Could you check a few things on this model? Use its own coordinates, in mm. Face numbers are marked on the shaded views. A direction names the side the tool comes from. Coordinates: 2 decimals unless noted, no trailing zeros. Loops run counter-clockwise (first coordinate to the right, second up) from the corner with the lowest first, then second, coordinate; pieces in that order, holes last. Notation, with made-up numbers: (1, 61) -> (59, 61) arc R37 ccw to (59, 98) -> close; hole circle Ø3 at (11.25, 64). An arc over 180 degrees is marked (long way). One line per question, with ' | ' between items.
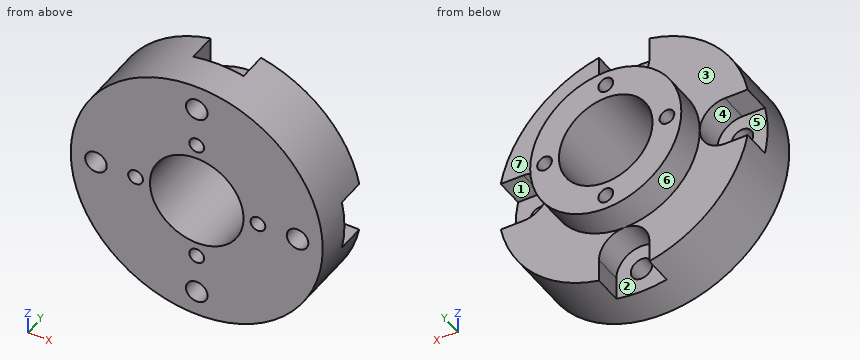
```python
from build123d import *

# Parameters (mm, degrees)
HOLE_WIZARD_4_1_4_1_1_D     = 4.1
HOLE_WIZARD_4_1_4_1_1_DEPTH = 26.501
HOLE_WIZARD_6_0_6_1_D       = 6
HOLE_WIZARD_6_0_6_1_DEPTH   = 18.001
CUT_EXTRUDE_1_DEPTH         = 8
PATTERN_CIRCULAR_1_COUNT    = 4


with BuildPart() as part:
    # Эскиз1 → Повернуть1 (revolve)
    with BuildSketch(Plane.XY):
        Polygon((-13, 0), (-13, 26.5), (-21, 26.5), (-21, 18), (-35, 18), (-35, 0), align=None)
    revolve(axis=Axis((0, 0, 0), (0, 1, 0)))

    # Диаметр отверстия Ø4.1 (4.1)1
    with Locations(Plane(origin=(0, 26.5, 0), x_dir=(1, 0, 0), z_dir=(0, 1, 0))):
        with Locations((17, 0)):
            hole_wizard_4_1_4_1_1 = Hole(HOLE_WIZARD_4_1_4_1_1_D / 2, depth=HOLE_WIZARD_4_1_4_1_1_DEPTH)

    # Диаметр отверстия Ø6.0 (6)1
    with Locations(Plane(origin=(0, 18, 0), x_dir=(1, 0, 0), z_dir=(0, 1, 0))):
        with Locations((28, 0)):
            hole_wizard_6_0_6_1 = Hole(HOLE_WIZARD_6_0_6_1_D / 2, depth=HOLE_WIZARD_6_0_6_1_DEPTH)

    # Эскиз4 → Вырез-Вытянуть1 (cut)
    with BuildSketch(Plane(origin=(0, 18, 0), x_dir=(1, 0, 0), z_dir=(0, 1, 0))):
        with BuildLine():
            Line((28, 7), (48, 7))
            Line((48, 7), (48, -7))
            Line((48, -7), (28, -7))
            ThreePointArc((28, -7), (21, 0), (28, 7))
        make_face()
    cut_extrude_1 = extrude(amount=-CUT_EXTRUDE_1_DEPTH, mode=Mode.SUBTRACT)

    # Круговой массив1: Диаметр отверстия Ø4.1 (4.1)1, Диаметр отверстия Ø6.0 (6)1, Вырез-Вытянуть1 ×4 about axis
    pattern_circular_1_axis = Axis((0, 0, 0), (0, 1, 0))
    for i in range(1, PATTERN_CIRCULAR_1_COUNT):
        add(hole_wizard_4_1_4_1_1.rotate(pattern_circular_1_axis, i * 360 / PATTERN_CIRCULAR_1_COUNT), mode=Mode.SUBTRACT)
        add(hole_wizard_6_0_6_1.rotate(pattern_circular_1_axis, i * 360 / PATTERN_CIRCULAR_1_COUNT), mode=Mode.SUBTRACT)
        add(cut_extrude_1.rotate(pattern_circular_1_axis, i * 360 / PATTERN_CIRCULAR_1_COUNT), mode=Mode.SUBTRACT)


solid = part.part
```
Q1. We'd pull the mould along Z, two halves only. Please class the marked faces 5, 6 and 7: released by +Z, released by -Z, zero draft, split by the parting line, or undercut.
Values follow:
face 5: undercut | face 6: split by the parting line | face 7: zero draft
Q2. Imagine slicing it at A-A on y = 2.75. Give the number of separate pieces and of enclosed holes in the cut face, plus the area to 3 significant figures.
Values follow:
separate pieces: 1 | enclosed holes: 9 | area: 3,150 mm2
Q3. For pin 1 (4 mm diameter, centred on x = 30.5, z = 2, fed in from +Y); pin 2 (3 mm diameter, centred on x = 32, y = 14.5, fed in from -Z); pin 3 (3 mm diameter, centred on x = -31.5, y = 15, fed in from -Z); pin 4 (3.5 mm diameter, centred on x = 0, z = -17, fed in from +Y), each with a flat end and sliding along its axis, tell me the tip position at first contact or that it passes through.
Values follow:
pin 1: stops at y = 10 | pin 2: stops at z = -17.17 | pin 3: stops at z = -18.03 | pin 4: passes through
Q4. Imagine slicing it at B-B on x = 9. Write out the boundary of the cut face in (y, z).
Values follow:
outline: (0, -33.82) -> (18, -33.82) -> (18, -18.97) -> (26.5, -18.97) -> (26.5, -9.38) -> (0, -9.38) -> close; (0, 9.38) -> (26.5, 9.38) -> (26.5, 18.97) -> (18, 18.97) -> (18, 33.82) -> (0, 33.82) -> close
Q5. Imagine slicing it at C-C on y = 21. Write out the boundary of the cut face in (x, z), plus the area to 3 significant figures.
Values follow:
outline: circle Ø42 at (0, 0); hole circle Ø4.1 at (-17, 0); hole circle Ø26 at (0, 0); hole circle Ø4.1 at (0, -17); hole circle Ø4.1 at (0, 17); hole circle Ø4.1 at (17, 0) | area: 802 mm2
Q6. Imagine slicing it at D-D on z = 10. Write out the boundary of the cut face in (x, y), plus the area to 3 significant figures.
Values follow:
outline: (-33.54, 0) -> (-8.31, 0) -> (-8.31, 26.5) -> (-18.47, 26.5) -> (-18.47, 18) -> (-33.54, 18) -> close; (8.31, 0) -> (33.54, 0) -> (33.54, 18) -> (18.47, 18) -> (18.47, 26.5) -> (8.31, 26.5) -> close | area: 1,080 mm2
Q7. For the marked faces 1, 2, 3 and 4, which set-ups out of +Z, -Z, +X, -X, +Y, -Y let a thin tool reach every point of the face, with its end or its side?
Values follow:
face 1: +X, +Y | face 2: -Z, +Y | face 3: +Z, -X, +Y | face 4: -X, +Y
Q8. Please list where these lines run through material, in increasing order: L1, parallel to Z at x = 28, y = 3; L2, parallel to X at y = 10.5, z = 18. Write a range as [from, to].
Values follow:
L1: z = [-21, -3], [3, 21] | L2: x = [-30.02, -1.79], [1.79, 30.02]
